Input: part model. Units: mm. Frame: model coordinates. A direction names the side the tool comes from. Give positions to 0.01 mm unless a question says otherwise; leave off trailing zeros. Use a Markdown table: item, result. Add a question column.
1. Set-up query: faces 5 (the flat face through (-92.7, 2.6, 0)), 6 (the cylindrical face through (-84.479, 0.987, 4.886)), 7 (the flat face through (-88.247, 0.13, 3.156)). Return all of +Z, -Z, +X, -X, +Y, -Y with unobstructed straight access to the full face (end or side cutting, diameter ignored); none if empty.
2. Material intervals for probe 1 along Z at (x, y) = (-92, 3); probe 2 along Z at (x, y) = (-85.85, 2.5); probe 3 along Z at (x, y) = (-90.65, 2.5), sorted ascending.
3. Mould query, pull axis Z, two halves, no side actions, for faces 1 (the flat face through (-87.014, 4.2, 4.5)), 2 (the flat face through (-100.114, 3, -3)), 3 (the flat face through (-92, 2, 9.1)), 4 (the flat face through (-82.014, 4, 6)). Classes: released by +Z, released by -Z, zero draft, split by the parting line, or undercut.
4. Section query A-A, the plane y = 2.5. Count the separate pieces of the cut face and the enclosed holes in it, plus the area to 3 significant figures.
5. Pin query (flat end, axial travel): pin 1 (5 mm diameter, centred on x = -84.5, y = 4, fed in from +Z); pin 2 (3 mm diameter, centred on x = -94.56, y = 2.5, fed in from +Z); pin 3 (1.9 mm diameter, centred on y = 2.5, z = 4.55, fed in from +X); pin 4 (2 mm diameter, centred on x = -88, y = 4.5, fed in from -Z). Return the tip coordinate at first contact, or that it passes through.
```python
from build123d import *

# Parameters (mm, degrees)
SKETCH1_R               = 4.55
SKETCH1_R_2             = 1.55
BOSS_EXTRUDE1_DEPTH     = 9.1
SKETCH2_R               = 1.55
BOSS_EXTRUDE2_DEPTH     = 3
SKETCH3_W               = 17.1
SKETCH3_H               = 9.1
BOSS_EXTRUDE3_DEPTH     = 3
CUT_EXTRUDE1_REACH      = 26.036
CUT_EXTRUDE1_END_RADIUS = 3.55
SKETCH4_R               = 1.55
SKETCH5_R               = 1.55
CUT_EXTRUDE2_DEPTH      = 2.5
CHAMFER1_SIZE           = 1
CHAMFER2_SIZE           = 3


with BuildPart() as part:
    # Sketch1 → Boss-Extrude1 (new body)
    # profile 1 of 3: a face of its own
    with BuildSketch(Plane.XY):
        with Locations((-94.564189657, 2.5)):
            Circle(SKETCH1_R)
        with Locations((-94.564189657, 2.5)):
            Circle(SKETCH1_R_2, mode=Mode.SUBTRACT)
    # profile 2 of 3: a face of its own
    with BuildSketch(Plane.XY):
        with BuildLine():
            ThreePointArc((-94.564189657, -2.05), (-99.114189657, 2.5), (-94.564189657, 7.05))
            Line((-94.564189657, 7.05), (-100.114189657, 7.05))
            Line((-100.114189657, 7.05), (-100.114189657, -2.05))
            Line((-100.114189657, -2.05), (-94.564189657, -2.05))
        make_face()
    # profile 3 of 3: a face of its own
    with BuildSketch(Plane.XY):
        with BuildLine():
            Line((-85.014189657, 7.05), (-94.564189657, 7.05))
            ThreePointArc((-94.564189657, 7.05), (-91.346853802, 5.717335854), (-90.014189657, 2.5))
            ThreePointArc((-90.014189657, 2.5), (-91.346853802, -0.717335854), (-94.564189657, -2.05))
            Line((-94.564189657, -2.05), (-85.014189657, -2.05))
            Line((-85.014189657, -2.05), (-85.014189657, 7.05))
        make_face()
    extrude(amount=BOSS_EXTRUDE1_DEPTH)



with BuildPart() as body_2:
    # Sketch2 → Boss-Extrude2 (new body)
    # profile 1 of 2: a face of its own
    with BuildSketch(Plane(origin=(0, 0, -5), x_dir=(-1, 0, 0), z_dir=(0, 0, -1))):
        with BuildLine():
            ThreePointArc((99.114189657, 2.5), (97.781525511, 5.717335854), (94.564189657, 7.05))
            ThreePointArc((94.564189657, 7.05), (90.014189657, 2.5), (94.564189657, -2.05))
            ThreePointArc((94.564189657, -2.05), (97.781525511, -0.717335854), (99.114189657, 2.5))
        make_face()
        with Locations(Location((94.564189657, 2.5, 0), (0, 0, 180))):
            Circle(SKETCH2_R, mode=Mode.SUBTRACT)
    # profile 2 of 2: a face of its own
    with BuildSketch(Plane(origin=(0, 0, -5), x_dir=(-1, 0, 0), z_dir=(0, 0, -1))):
        with BuildLine():
            Line((100.114189657, -2.05), (100.114189657, 7.05))
            Line((100.114189657, 7.05), (94.564189657, 7.05))
            ThreePointArc((94.564189657, 7.05), (97.781525511, 5.717335854), (99.114189657, 2.5))
            ThreePointArc((99.114189657, 2.5), (97.781525511, -0.717335854), (94.564189657, -2.05))
            Line((94.564189657, -2.05), (100.114189657, -2.05))
        make_face()
    extrude(amount=BOSS_EXTRUDE2_DEPTH)


with BuildPart() as part_1:
    add(part.part)

    add(body_2.part)  # Boss-Extrude3 merges body 2
    # Sketch3 → Boss-Extrude3 (add)
    with BuildSketch(Plane.ZY.offset(100.114189657)):
        with Locations((0.55, 2.5)):
            Rectangle(SKETCH3_W, SKETCH3_H)
    extrude(amount=BOSS_EXTRUDE3_DEPTH)

    # Loft1: read off the stored shape, not the designer's step
    # Loft1: loft between two sections, ruled curve by curve
    loft1_from = [
        Edge.make_bspline([(-85.014189657, -2.05, 9.1), (-85.014189657, -2.05, 8.341666667), (-85.014189657, -2.05, 7.583333333), (-85.014189657, -2.05, 6.066666667), (-85.014189657, -2.05, 5.308333333), (-85.014189657, -2.05, 3.791666667), (-85.014189657, -2.05, 3.033333333), (-85.014189657, -2.05, 1.516666667), (-85.014189657, -2.05, 0.758333333), (-85.014189657, -2.05, 0)], [0, 0, 0, 0, 0.25, 0.25, 0.5, 0.5, 0.75, 0.75, 1, 1, 1, 1], 3),
        Edge.make_bspline([(-85.014189657, -2.05, 0), (-85.014189657, -1.291666667, 0), (-85.014189657, -0.533333333, 0), (-85.014189657, 0.983333333, 0), (-85.014189657, 1.741666667, 0), (-85.014189657, 3.258333333, 0), (-85.014189657, 4.016666667, 0), (-85.014189657, 5.533333333, 0), (-85.014189657, 6.291666667, 0), (-85.014189657, 7.05, 0)], [0, 0, 0, 0, 0.25, 0.25, 0.5, 0.5, 0.75, 0.75, 1, 1, 1, 1], 3),
        Edge.make_bspline([(-85.014189657, 7.05, 9.1), (-85.014189657, 6.291666667, 9.1), (-85.014189657, 5.533333333, 9.1), (-85.014189657, 4.016666667, 9.1), (-85.014189657, 3.258333333, 9.1), (-85.014189657, 1.741666667, 9.1), (-85.014189657, 0.983333333, 9.1), (-85.014189657, -0.533333333, 9.1), (-85.014189657, -1.291666667, 9.1), (-85.014189657, -2.05, 9.1)], [0, 0, 0, 0, 0.25, 0.25, 0.5, 0.5, 0.75, 0.75, 1, 1, 1, 1], 3),
        Edge.make_bspline([(-85.014189657, 7.05, 0), (-85.014189657, 7.05, 0.758333333), (-85.014189657, 7.05, 1.516666667), (-85.014189657, 7.05, 3.033333333), (-85.014189657, 7.05, 3.791666667), (-85.014189657, 7.05, 5.308333333), (-85.014189657, 7.05, 6.066666667), (-85.014189657, 7.05, 7.583333333), (-85.014189657, 7.05, 8.341666667), (-85.014189657, 7.05, 9.1)], [0, 0, 0, 0, 0.25, 0.25, 0.5, 0.5, 0.75, 0.75, 1, 1, 1, 1], 3),
    ]
    loft1_to = [
        Edge.make_bspline([(-82.014189657, 0.378679656, 6.671320344), (-82.014189657, 0.128679656, 6.421320344), (-82.014189657, -0.095475789, 6.106038327), (-82.014189657, -0.410975479, 5.377025758), (-82.014189657, -0.5, 4.964213562), (-82.014189657, -0.5, 4.135786438), (-82.014189657, -0.410975479, 3.722974242), (-82.014189657, -0.095475789, 2.993961673), (-82.014189657, 0.128679656, 2.678679656), (-82.014189657, 0.378679656, 2.428679656)], [0, 0, 0, 0, 0.25, 0.25, 0.5, 0.5, 0.75, 0.75, 1, 1, 1, 1], 3),
        Edge.make_bspline([(-82.014189657, 0.378679656, 2.428679656), (-82.014189657, 0.628679656, 2.178679656), (-82.014189657, 0.943961673, 1.954524211), (-82.014189657, 1.672974242, 1.639024521), (-82.014189657, 2.085786438, 1.55), (-82.014189657, 2.914213562, 1.55), (-82.014189657, 3.327025758, 1.639024521), (-82.014189657, 4.056038327, 1.954524211), (-82.014189657, 4.371320344, 2.178679656), (-82.014189657, 4.621320344, 2.428679656)], [0, 0, 0, 0, 0.25, 0.25, 0.5, 0.5, 0.75, 0.75, 1, 1, 1, 1], 3),
        Edge.make_bspline([(-82.014189657, 4.621320344, 6.671320344), (-82.014189657, 4.371320344, 6.921320344), (-82.014189657, 4.056038327, 7.145475789), (-82.014189657, 3.327025758, 7.460975479), (-82.014189657, 2.914213562, 7.55), (-82.014189657, 2.085786438, 7.55), (-82.014189657, 1.672974242, 7.460975479), (-82.014189657, 0.943961673, 7.145475789), (-82.014189657, 0.628679656, 6.921320344), (-82.014189657, 0.378679656, 6.671320344)], [0, 0, 0, 0, 0.25, 0.25, 0.5, 0.5, 0.75, 0.75, 1, 1, 1, 1], 3),
        Edge.make_bspline([(-82.014189657, 4.621320344, 2.428679656), (-82.014189657, 4.871320344, 2.678679656), (-82.014189657, 5.095475789, 2.993961673), (-82.014189657, 5.410975479, 3.722974242), (-82.014189657, 5.5, 4.135786438), (-82.014189657, 5.5, 4.964213562), (-82.014189657, 5.410975479, 5.377025758), (-82.014189657, 5.095475789, 6.106038327), (-82.014189657, 4.871320344, 6.421320344), (-82.014189657, 4.621320344, 6.671320344)], [0, 0, 0, 0, 0.25, 0.25, 0.5, 0.5, 0.75, 0.75, 1, 1, 1, 1], 3),
    ]
    loft1 = Solid(Shell([*[Face.make_surface_from_curves(loft1_from[k], loft1_to[k]) for k in range(4)], Face(Wire(loft1_from)), Face(Wire(loft1_to))]))
    add(loft1)

    # Cut-Extrude1: up to this cylinder (the profile starts outside it)
    cut_extrude1_end = Plane(origin=(-94.564189657, 2.5, 4.55), z_dir=(0, 0, -1)) * Cylinder(CUT_EXTRUDE1_END_RADIUS, 60.172, mode=Mode.PRIVATE)
    # Sketch4 → Cut-Extrude1 (cut, up to the surface)
    with BuildSketch(Plane(origin=(-82.014189657, 0, 0), x_dir=(0, 0, -1), z_dir=(1, 0, 0)), mode=Mode.PRIVATE) as cut_extrude1_sk1:
        with Locations((-4.55, 2.5)):
            Circle(SKETCH4_R)
    cut_extrude1_tool1 = extrude(cut_extrude1_sk1.sketch, amount=-CUT_EXTRUDE1_REACH, mode=Mode.PRIVATE) - cut_extrude1_end
    add(cut_extrude1_tool1.solids().sort_by_distance((-82.01419, 2.5, 4.55))[0], mode=Mode.SUBTRACT)

    # Sketch5 → Cut-Extrude2 (cut)
    # profile 1 of 2: a face of its own
    with BuildSketch(Plane.ZY.offset(87.014189657)):
        Polygon((4.55, 5.675426481), (7.3, 4.08771324), (7.3, 7.05), (1.8, 7.05), (1.8, 4.08771324), align=None)
    # profile 2 of 2: a face of its own
    with BuildSketch(Plane.ZY.offset(87.014189657)):
        Polygon((7.3, 0.91228676), (7.3, 4.08771324), (4.55, 5.675426481), (1.8, 4.08771324), (1.8, 0.91228676), (4.55, -0.675426481), align=None)
        with Locations(Location((4.55, 2.5, 0), (0, 0, 180))):
            Circle(SKETCH5_R, mode=Mode.SUBTRACT)
    extrude(amount=CUT_EXTRUDE2_DEPTH, mode=Mode.SUBTRACT)

    # Chamfer1
    chamfer1_edges = [part_1.edges().sort_by_distance(p)[0] for p in [
        (-87.014189657, 7.05, 4.55),
        (-88.264189657, 7.05, 7.3),
        (-88.264189657, 7.05, 1.8),
        (-89.514189657, 7.05, 4.55),
    ]]
    chamfer(chamfer1_edges, length=CHAMFER1_SIZE)

    # Chamfer2
    chamfer2_edges = [part_1.edges().sort_by_distance(p)[0] for p in [
        (-103.114189657, 2.5, 9.1),
    ]]
    chamfer(chamfer2_edges, length=CHAMFER2_SIZE)


solid = part_1.part
```
Result sheet:
| question | item | result |
|---|---|---|
| 1 | face 5 | +X, +Y, -Y |
| 1 | face 6 | +X |
| 1 | face 7 | +Y |
| 2 | probe 1 | z = -8 to -5, 0 to 9.1 |
| 2 | probe 2 | z = 0 to 3, 6.1 to 9.1 |
| 2 | probe 3 | z = -8 to -5, 0 to 3, 6.1 to 9.1 |
| 3 | face 1 | undercut |
| 3 | face 2 | undercut |
| 3 | face 3 | released by +Z |
| 3 | face 4 | zero draft |
| 4 | separate pieces | 3 |
| 4 | enclosed holes | 0 |
| 4 | area | 166 mm² |
| 5 | pin 1 | stops at z = 9.1 |
| 5 | pin 2 | passes through |
| 5 | pin 3 | stops at x = -91.01 |
| 5 | pin 4 | stops at z = 0 |
